```python
from build123d import *

# Parameters (mm, degrees)
BOSS_EXTRUDE1_DEPTH      = 1.5875
BOSS_EXTRUDE1_DEPTH_BACK = 1.5875
SKETCH1_W                = 75
SKETCH1_H                = 60
CUT_EXTRUDE1_DEPTH       = 49.049663435
CUT_EXTRUDE1_DEPTH_BACK  = 49.049663435
SKETCH2_R                = 2.7
CUT_EXTRUDE2_DEPTH       = 49.049663435
CUT_EXTRUDE2_DEPTH_BACK  = 49.049663435
SKETCH3_R                = 10.668
SKETCH3_R_2              = 1.5875


with BuildPart() as part:
    # Sketch1 → Boss-Extrude1 (new, two sides: drawn at the far end of the back side and taken through both)
    with BuildSketch(Plane(origin=(0, 0, 0), x_dir=(0, 0, -1), z_dir=(1, 0, 0)).offset(-BOSS_EXTRUDE1_DEPTH_BACK)):
        Rectangle(SKETCH1_W, SKETCH1_H)
    extrude(amount=BOSS_EXTRUDE1_DEPTH + BOSS_EXTRUDE1_DEPTH_BACK)

    # Sketch2 → Cut-Extrude1 (cut, two sides: drawn at the far end of the back side and taken through both)
    with BuildSketch(Plane(origin=(0, 0, 0), x_dir=(0, 0, -1), z_dir=(1, 0, 0)).offset(-CUT_EXTRUDE1_DEPTH_BACK)):
        with Locations((-31.05, 23.55)):
            Circle(SKETCH2_R)
        with Locations(Location((31.05, 23.55, 0), (0, 0, 180))):
            Circle(SKETCH2_R)
        with Locations((31.05, -23.55)):
            Circle(SKETCH2_R)
        with Locations(Location((-31.05, -23.55, 0), (0, 0, 180))):
            Circle(SKETCH2_R)
    extrude(amount=CUT_EXTRUDE1_DEPTH + CUT_EXTRUDE1_DEPTH_BACK, mode=Mode.SUBTRACT)

    # Sketch3 → Cut-Extrude2 (cut, two sides: drawn at the far end of the back side and taken through both)
    with BuildSketch(Plane(origin=(0, 0, 0), x_dir=(0, 0, -1), z_dir=(1, 0, 0)).offset(-CUT_EXTRUDE2_DEPTH_BACK)):
        Circle(SKETCH3_R)
        with Locations((-10.7188, 10.7188)):
            Circle(SKETCH3_R_2)
        with Locations((10.7188, 10.7188)):
            Circle(SKETCH3_R_2)
        with Locations((10.7188, -10.7188)):
            Circle(SKETCH3_R_2)
        with Locations((-10.7188, -10.7188)):
            Circle(SKETCH3_R_2)
    extrude(amount=CUT_EXTRUDE2_DEPTH + CUT_EXTRUDE2_DEPTH_BACK, mode=Mode.SUBTRACT)


solid = part.part
```
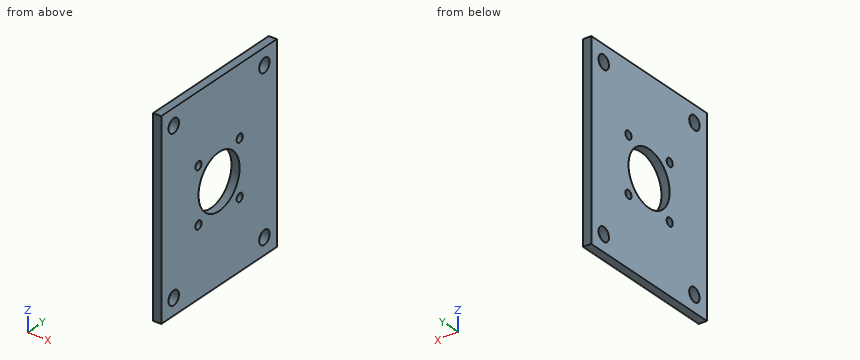
Could you check a few things on this model? Use its own coordinates, in mm. Give positions to 0.01 mm unless a question says otherwise; leave off trailing zeros. Loops run counter-clockwise (first coordinate to the right, second up) from the corner with the lowest first, then second, coordinate; pieces in that order, holes last. Notation, with made-up numbers: (46.25, 88) - (68.25, 88) arc R21 ccw to (68.25, 113) - close; hole circle Ø8 at (18.25, -40). An arc over 180 degrees is marked (long way). Use one line per item in the form item = value.
1. I'm going to push flat-ended pins straight in: pin 1 Ø19 at (y, z) = (0, 0) entering from -X; pin 2 Ø7 at (y, z) = (-23.55, -31.05) entering from -X. Where does each tip first touch, or does it pass through?
Response values:
pin_1 = through
pin_2 = -1.59
2. I want a section at B-B (z = 31.05). Please give me the cut outline in (x, y).
Response values:
outline = (-1.59, -30) - (1.59, -30) - (1.59, -26.25) - (-1.59, -26.25) - close; (-1.59, -20.85) - (1.59, -20.85) - (1.59, 20.85) - (-1.59, 20.85) - close; (-1.59, 26.25) - (1.59, 26.25) - (1.59, 30) - (-1.59, 30) - close
3. I need wall thicknesses on probe 1 along Y at (x, z) = (0.8, 31.05); probe 2 along Z at (x, y) = (0.3, 0); probe 3 along Z at (x, y) = (-1.2, -5.5). Which ranges of each line are inside material? Lowest first, please.
Response values:
probe_1 = -30 to -26.25, -20.85 to 20.85, 26.25 to 30
probe_2 = -37.5 to -10.67, 10.67 to 37.5
probe_3 = -37.5 to -9.14, 9.14 to 37.5
4. I want a section at C-C (y = 23.55). Please give me the cut outline in (x, z), and give its area (3 significant figures).
Response values:
outline = (-1.59, -37.5) - (1.59, -37.5) - (1.59, -33.75) - (-1.59, -33.75) - close; (-1.59, -28.35) - (1.59, -28.35) - (1.59, 28.35) - (-1.59, 28.35) - close; (-1.59, 33.75) - (1.59, 33.75) - (1.59, 37.5) - (-1.59, 37.5) - close
area = 204 mm²
5. I want a section at A-A (y = 0). Please give me the cut outline in (x, z).
Response values:
outline = (-1.59, -37.5) - (1.59, -37.5) - (1.59, -10.67) - (-1.59, -10.67) - close; (-1.59, 10.67) - (1.59, 10.67) - (1.59, 37.5) - (-1.59, 37.5) - close
6. I want a section at D-D (z = 0). Please give me the cut outline in (x, y).
Response values:
outline = (-1.59, -30) - (1.59, -30) - (1.59, -10.67) - (-1.59, -10.67) - close; (-1.59, 10.67) - (1.59, 10.67) - (1.59, 30) - (-1.59, 30) - close
